Verification items for this drawing (mm, ordinates from the low corner). A direction names the side the tool comes from. Give positions to 0.01 mm unless a question says otherwise; leave off trailing zeros. Loops run counter-clockwise (first coordinate to the right, second up) from the corner with the lowest first, then second, coordinate; pieces in that order, holes last. Notation, with made-up numbers: M 45,-25 L 76,-25 A18 cw 76,9 Z; hole C 41,87.5 d5. An arc over 180 degrees is marked long. Write each question's results on one line, items separated by ' | '. Start each with the question number.
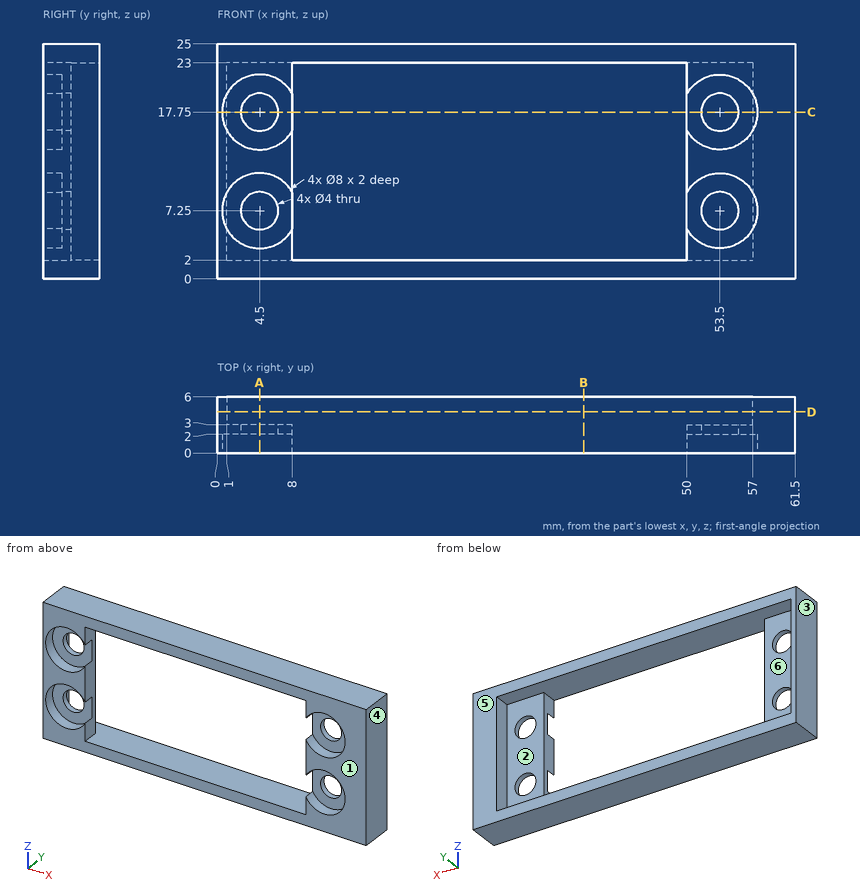
1. Thickness scan on probe 1 along Z at (x, y) = (53.5, 2.45); probe 2 along Z at (x, y) = (4.5, 1.05); probe 3 along Z at (x, y) = (23, 2.25). Record the ranges inside material, lowest first.
2. Section check D-D, the plane y = 4.4. Record the boundary of the cut face in (x, z).
3. Release check for a two-part mould opening along X. For the marked faces 1, 2, 3 and 4 record: released by +X, released by -X, zero draft, split by the parting line, or undercut.
4. Depth check by flat-ended pin: pin 1 Ø2.5 at (x, z) = (53.5, 17.75) entering from -Y; pin 2 Ø6.5 at (x, z) = (4.5, 7.25) entering from +Y; pin 3 Ø4.5 at (x, z) = (4.5, 17.75) entering from -Y. Enter the tip coordinate at first touch or a pass-through.
5. Section check B-B, the plane x = 39. Record the boundary of the cut face in (y, z).
6. Section check C-C, the plane z = 17.75. Record the boundary of the cut face in (x, y), plus the area to 3 significant figures.
7. Set-up check for the marked faces 5 and 6: record each of +Z, -Z, +X, -X, +Y, -Y from which the full face is reachable in a straight line by a thin tool's end or side.
8. Section check A-A, the plane x = 4.5. Record the boundary of the cut face in (y, z), plus the area to 3 significant figures.
Filled sheet:
1) probe 1: 0 to 5.25, 9.25 to 15.75, 19.75 to 25 | probe 2: 0 to 3.25, 11.25 to 13.75, 21.75 to 25 | probe 3: 0 to 2, 23 to 25
2) outline: M 0,0 L 61.5,0 L 61.5,25 L 0,25 Z; hole M 1,2 L 57,2 L 57,23 L 1,23 Z
3) face 1: zero draft | face 2: undercut | face 3: released by -X | face 4: released by +X
4) pin 1: through | pin 2: y = 3 | pin 3: y = 2
5) outline: M 0,0 L 6,0 L 6,2 L 0,2 Z; M 0,23 L 6,23 L 6,25 L 0,25 Z
6) outline: M 0,0 L 0.5,0 L 0.5,2 L 2.5,2 L 2.5,3 L 1,3 L 1,6 L 0,6 Z; M 6.5,2 L 8,2 L 8,3 L 6.5,3 Z; M 50,2 L 51.5,2 L 51.5,3 L 50,3 Z; M 55.5,2 L 57.5,2 L 57.5,0 L 61.5,0 L 61.5,6 L 57,6 L 57,3 L 55.5,3 Z | area: 37.0 mm2
7) face 5: +Z, -Z, +X, -X, +Y | face 6: +Y
8) outline: M 0,0 L 6,0 L 6,2 L 3,2 L 3,5.25 L 2,5.25 L 2,3.25 L 0,3.25 Z; M 0,11.25 L 2,11.25 L 2,9.25 L 3,9.25 L 3,15.75 L 2,15.75 L 2,13.75 L 0,13.75 Z; M 0,21.75 L 2,21.75 L 2,19.75 L 3,19.75 L 3,23 L 6,23 L 6,25 L 0,25 Z | area: 47.0 mm2
